```python
from build123d import *

# Parameters (mm, degrees)
F0_W         = 200
F0_H         = 150
F0_R         = 12.0683860383
F0_R_2       = 60
F1_DEPTH     = 80
F2_DEPTH     = 138
F3_C1_SIZE2  = 12
F3_C1_SIZE   = 11
F3_C2_SIZE2  = 12
F3_C2_SIZE   = 11
F3_C3_SIZE2  = 12
F3_C3_SIZE   = 11
F3_C4_SIZE2  = 12
F3_C4_SIZE   = 11
F4_DEPTH     = 50
F5_R         = 49.7327993849
F7_DEPTH     = 40
F8_DEPTH     = 20
F11_T2_ANGLE = 180


# Not quite as in the source:
# - a fillet or chamfer that OpenCascade refuses, or shapes differently, is made with other operations: its cross-section is extruded or revolved along the edge and cut away or added


with BuildPart() as f1:
    # F0 (on Front) → F1 (new body)
    with BuildSketch(Plane.XZ):
        Rectangle(F0_W, F0_H)
        with Locations((-81.3817187923, -60)):
            Circle(F0_R, mode=Mode.SUBTRACT)
        with Locations((81.3817187923, -60)):
            Circle(F0_R, mode=Mode.SUBTRACT)
        with Locations((-81.3817187923, 60)):
            Circle(F0_R, mode=Mode.SUBTRACT)
        Circle(F0_R_2, mode=Mode.SUBTRACT)
        with Locations((81.3817187923, 60)):
            Circle(F0_R, mode=Mode.SUBTRACT)
        Circle(F0_R_2)
        with Locations((81.3817187923, -60)):
            Circle(F0_R)
        with Locations((-81.3817187923, 60)):
            Circle(F0_R)
        with Locations((-81.3817187923, -60)):
            Circle(F0_R)
        with Locations((81.3817187923, 60)):
            Circle(F0_R)
    extrude(amount=-F1_DEPTH)

    # F0 (on Front) → F2 (join)
    with BuildSketch(Plane.XZ):
        with Locations((-81.3817187923, 60)):
            Circle(F0_R)
        with Locations((81.3817187923, 60)):
            Circle(F0_R)
        with Locations((81.3817187923, -60)):
            Circle(F0_R)
        with Locations((-81.3817187923, -60)):
            Circle(F0_R)
    extrude(amount=F2_DEPTH)

    # F3: chamfer of 12 x 11 on 4 edges, made by hand

    # F3_c1
    f3_c1_edges = [f1.edges().sort_by_distance(p)[0] for p in [
        (-93.4501048306, -138, -60),
    ]]
    f3_c1_side = f1.faces().sort_by_distance((-93.4501048306, -137.78, -60))[0]
    chamfer(f3_c1_edges, length=F3_C1_SIZE, length2=F3_C1_SIZE2, reference=f3_c1_side)

    # F3_c2
    f3_c2_edges = [f1.edges().sort_by_distance(p)[0] for p in [
        (69.313332754, -138, -60),
    ]]
    f3_c2_side = f1.faces().sort_by_distance((69.313332754, -137.78, -60))[0]
    chamfer(f3_c2_edges, length=F3_C2_SIZE, length2=F3_C2_SIZE2, reference=f3_c2_side)

    # F3_c3
    f3_c3_edges = [f1.edges().sort_by_distance(p)[0] for p in [
        (-93.4501048306, -138, 60),
    ]]
    f3_c3_side = f1.faces().sort_by_distance((-93.4501048306, -137.78, 60))[0]
    chamfer(f3_c3_edges, length=F3_C3_SIZE, length2=F3_C3_SIZE2, reference=f3_c3_side)

    # F3_c4
    f3_c4_edges = [f1.edges().sort_by_distance(p)[0] for p in [
        (69.313332754, -138, 60),
    ]]
    f3_c4_side = f1.faces().sort_by_distance((69.313332754, -137.78, 60))[0]
    chamfer(f3_c4_edges, length=F3_C4_SIZE, length2=F3_C4_SIZE2, reference=f3_c4_side)

    # F0 (on Front) → F4 (join)
    with BuildSketch(Plane.XZ):
        Circle(F0_R_2)
    extrude(amount=F4_DEPTH)

    # F5
    f5_edges = [f1.edges().sort_by_distance(p)[0] for p in [
        (-60, -50, 0),
    ]]
    fillet(f5_edges, radius=F5_R)

    # F6 (on face) → F7 (join)
    with BuildSketch(Plane(origin=(0, 0, -75), x_dir=(1, 0, 0), z_dir=(0, 0, -1))):
        with BuildLine():
            ThreePointArc((-68.6766029522, -11.3233970478), (-71.9931491676, -3.316546203), (-80.0000000175, 0))
            ThreePointArc((-80.0000000175, 0), (-88.0068508448, -3.3165462154), (-91.3233970478, -11.3233970478))
            Line((-91.3233970478, -11.3233970478), (-91.3233970478, -17.7343630829))
            Line((-91.3233970478, -17.7343630829), (-100, -22.6467940956))
            Line((-100, -22.6467940956), (-100, -80))
            Line((-100, -80), (-60, -80))
            Line((-60, -80), (-60, -22.6467940956))
            Line((-60, -22.6467940956), (-68.6766029522, -17.7343630829))
            Line((-68.6766029522, -17.7343630829), (-68.6766029522, -11.3233970478))
        make_face()
        with BuildLine():
            Line((68.6766029522, -17.7343630829), (60, -22.6467940956))
            Line((60, -22.6467940956), (60, -80))
            Line((60, -80), (100, -80))
            Line((100, -80), (100, -22.6467940956))
            Line((100, -22.6467940956), (91.3233970478, -17.7343630829))
            Line((91.3233970478, -17.7343630829), (91.3233970478, -11.3233970478))
            ThreePointArc((91.3233970478, -11.3233970478), (88.0068508386, -3.3165462092), (80, 0))
            ThreePointArc((80, 0), (71.9931491614, -3.3165462092), (68.6766029522, -11.3233970478))
            Line((68.6766029522, -11.3233970478), (68.6766029522, -17.7343630829))
        make_face()
    extrude(amount=F7_DEPTH)

    # F6 (on face) → F8 (cut)
    with BuildSketch(Plane(origin=(0, 0, -75), x_dir=(1, 0, 0), z_dir=(0, 0, -1))):
        with BuildLine():
            ThreePointArc((60, -80), (0, -20), (-60, -80))
            Line((-60, -80), (60, -80))
        make_face()
    extrude(amount=-F8_DEPTH, mode=Mode.SUBTRACT)

    # F9 (on face) → F10 (revolve)
    with BuildSketch(Plane.YZ.offset(100)):
        with BuildLine():
            Line((80, 0), (0, 0))
            Line((0, 0), (0, -20))
            ThreePointArc((0, -20), (7.7276234195, -33.4243037519), (12.4269118533, -48.1838695705))
            Line((12.4269118533, -48.1838695705), (80, -48.1838695705))
            Line((80, -48.1838695705), (80, 0))
        make_face()
    revolve(axis=Axis((100, 40, 0), (0, 1, 0)))

    # F11: fillet of radius 5 on 1 edges, made by hand

    # F11_s1 → F11_t2 (revolve, cut)
    with BuildSketch(Plane.YZ.offset(100)):
        with BuildLine():
            ThreePointArc((0, 18.4024363766), (0.2292975701, 19.8992323966), (0.8961593302, 21.2587437405))
            ThreePointArc((0.8961593302, 21.2587437405), (0.451433447, 20.6269841539), (0, 20))
            Line((0, 20), (0, 18.4024363766))
        make_face()
    revolve(axis=Axis((100, 0, 0), (0, 1, 0)), revolution_arc=F11_T2_ANGLE, mode=Mode.SUBTRACT)


solid = f1.part
```
Could you check a few things on this model? Use its own coordinates, in mm. A direction names the side the tool comes from. Round coordinates to 2 decimals unless told otherwise and drop trailing zeros. Write each loop counter-clockwise with the first axis right and the second up, starting at its lowest first coordinate (ties: lowest second). Pieces come first, ordered by that corner, then holes.
(1) Which directions (+Z, -Z, +X, -X, +Y, -Y) give clear straight access to the entire face, cutting with the end or side of a thin tool? Please do faces 5 (the face through (60, 51, -95)), 6 (the face through (-65, 0, -1)), 7 (the face through (91.323, 15, -95)), 8 (the face through (-91.323, 14, -95)), 9 (the face through (-68.677, 15, -95)).
Findings below:
face 5: -Z, +Y, -Y
face 6: -Y
face 7: -Z, +X, -Y
face 8: -Z, -X, -Y
face 9: -Z, -Y
(2) Thinking about a two-plate mould opening in Z: for faces 1 (the face through (84.45, -135.02, -61.27)), 2 (the face through (68.677, 14, -95)), 3 (the face through (0, 16, -75)), 4 (the face through (-1, 39, 75)), which applies, +Z half, -Z half, draft (parallel to the pull), parting line (faces both ways), or undercut?
Findings below:
face 1: undercut
face 2: draft
face 3: -Z half
face 4: +Z half
(3) For pin 1 (1.9 mm diameter, centred on y = 15, z = -95.5, fed in from +X); pin 2 (24 mm diameter, centred on x = -15, y = 50, fed in from -Z); pin 3 (5 mm diameter, centred on y = 15.5, z = -88.5, fed in from -X), each with a flat end and sliding along its axis, tell me the tip position at first contact or that it passes through.
Findings below:
pin 1: stops at x = 91.32
pin 2: stops at z = -55
pin 3: stops at x = -91.79
(4) If I drill on probe 1 along X at (y, z) = (-124, 59); probe 2 along X at (y, z) = (26, -96); probe 3 along Y at (x, z) = (71, 7.5), over which ranges is the centre line in solid material (lowest first)?
Findings below:
probe 1: x = -93.41 to -69.35, 69.35 to 93.41
probe 2: x = -100 to -60, 60 to 100
probe 3: y = 0 to 80
(5) Suppose I cut it at B-B on y = 44. Write out the boundary of the cut face in (x, z).
Findings below:
outline: (-100, -115) - (-60, -115) - (-60, -75) - (-48, -75) - (-48, -55) - (48, -55) - (48, -75) - (60, -75) - (60, -115) - (100, -115) - (100, -48.18) arc R48.18 ccw to (100, 48.18) - (100, 75) - (-100, 75) - close
(6) Suppose I cut it at A-A on z = -80. Write out the boundary of the cut face in (x, y).
Findings below:
outline: (-100, 22.65) - (-91.32, 17.73) - (-91.32, 11.32) arc R11.32 ccw to (-68.68, 11.32) - (-68.68, 17.73) - (-60, 22.65) - (-60, 80) - (-100, 80) - close; (60, 22.65) - (68.68, 17.73) - (68.68, 11.32) arc R11.32 ccw to (91.32, 11.32) - (91.32, 17.73) - (100, 22.65) - (100, 80) - (60, 80) - close
